Can you work these out from the model? Positions are in its coordinate system, mm. A direction names the side the tool comes from. Coordinates: 2 decimals unless noted, no trailing zeros. Write each loop counter-clockwise with the first axis right and the second up, starting at its lowest first coordinate (ties: lowest second). Pieces come first, ordered by that corner, then holes. Notation, with made-up numbers: (57, -9.75) -> (91, -9.75) arc R19 ccw to (91, 16.25) -> close; hole circle Ø6 at (42, -26.5). An arc over 180 degrees is marked (long way). Use one line per item in the form item = value.
```python
from build123d import *

# Parameters (mm, degrees)
EXTRUDE_1_DEPTH              = 4
HOLE_WIZARD_M5_1_D           = 8
HOLE_WIZARD_M5_1_DEPTH       = 12.4
HOLE_WIZARD_M5_1_CBORE_D     = 9.5
HOLE_WIZARD_M5_1_CBORE_DEPTH = 0.9
HOLE_WIZARD_M5_1_TIP         = 2.403442476
HOLE_WIZARD_M5_2_D           = 8
HOLE_WIZARD_M5_2_DEPTH       = 12.4
HOLE_WIZARD_M5_2_CBORE_D     = 9.5
HOLE_WIZARD_M5_2_CBORE_DEPTH = 0.9
HOLE_WIZARD_M5_2_TIP         = 2.403442476


with BuildPart() as part:
    # 草图2 → 凸台-拉伸1 (new body)
    with BuildSketch(Plane(origin=(0, 0, 0), x_dir=(1, 0, 0), z_dir=(0, 1, 0))):
        with BuildLine():
            Line((20, 21.641016151), (28.741669751, 6.5))
            Line((28.741669751, 6.5), (40, 6.5))
            ThreePointArc((40, 6.5), (43.25, 5.629165125), (45.629165125, 3.25))
            Line((45.629165125, 3.25), (25.629165125, 37.891016151))
            ThreePointArc((25.629165125, 37.891016151), (26.5, 34.641016151), (25.629165125, 31.391016151))
            Line((25.629165125, 31.391016151), (20, 21.641016151))
        make_face()
        with BuildLine():
            Line((28.741669751, 6.5), (11.258330249, 6.5))
            Line((11.258330249, 6.5), (5.629165125, -3.25))
            ThreePointArc((5.629165125, -3.25), (3.25, -5.629165125), (0, -6.5))
            Line((0, -6.5), (40, -6.5))
            ThreePointArc((40, -6.5), (36.75, -5.629165125), (34.370834875, -3.25))
            Line((34.370834875, -3.25), (28.741669751, 6.5))
        make_face()
        with BuildLine():
            Line((40, 6.5), (28.741669751, 6.5))
            Line((28.741669751, 6.5), (34.370834875, -3.25))
            ThreePointArc((34.370834875, -3.25), (36.75, -5.629165125), (40, -6.5))
            ThreePointArc((40, -6.5), (45.629165125, -3.25), (45.629165125, 3.25))
            ThreePointArc((45.629165125, 3.25), (43.25, 5.629165125), (40, 6.5))
        make_face()
        with BuildLine():
            ThreePointArc((-5.629165125, 3.25), (-3.25, 5.629165125), (0, 6.5))
            Line((0, 6.5), (11.258330249, 6.5))
            Line((11.258330249, 6.5), (20, 21.641016151))
            Line((20, 21.641016151), (14.370834875, 31.391016151))
            ThreePointArc((14.370834875, 31.391016151), (13.5, 34.641016151), (14.370834875, 37.891016151))
            Line((14.370834875, 37.891016151), (-5.629165125, 3.25))
        make_face()
        with BuildLine():
            Line((14.370834875, 31.391016151), (20, 21.641016151))
            Line((20, 21.641016151), (25.629165125, 31.391016151))
            ThreePointArc((25.629165125, 31.391016151), (26.5, 34.641016151), (25.629165125, 37.891016151))
            ThreePointArc((25.629165125, 37.891016151), (20, 41.141016151), (14.370834875, 37.891016151))
            ThreePointArc((14.370834875, 37.891016151), (13.5, 34.641016151), (14.370834875, 31.391016151))
        make_face()
        with BuildLine():
            Line((11.258330249, 6.5), (0, 6.5))
            ThreePointArc((0, 6.5), (-3.25, 5.629165125), (-5.629165125, 3.25))
            ThreePointArc((-5.629165125, 3.25), (-5.629165125, -3.25), (0, -6.5))
            ThreePointArc((0, -6.5), (3.25, -5.629165125), (5.629165125, -3.25))
            Line((5.629165125, -3.25), (11.258330249, 6.5))
        make_face()
        Polygon((20, 21.641016151), (11.258330249, 6.5), (28.741669751, 6.5), align=None)
    extrude(amount=EXTRUDE_1_DEPTH)

    # M5 六角头螺栓的柱形沉头孔1
    with Locations(Plane(origin=(0, 4, 0), x_dir=(1, 0, 0), z_dir=(0, 1, 0))):
        with Locations((0, 0)):
            CounterBoreHole(HOLE_WIZARD_M5_1_D / 2, HOLE_WIZARD_M5_1_CBORE_D / 2, HOLE_WIZARD_M5_1_CBORE_DEPTH, depth=HOLE_WIZARD_M5_1_DEPTH)
            with Locations((0, 0, -(HOLE_WIZARD_M5_1_DEPTH + HOLE_WIZARD_M5_1_TIP / 2))):  # 118° drill point
                Cone(0, HOLE_WIZARD_M5_1_D / 2, HOLE_WIZARD_M5_1_TIP, mode=Mode.SUBTRACT)

    # M5 六角头螺栓的柱形沉头孔2
    with Locations(Plane(origin=(0, 0, 0), x_dir=(-1, 0, 0), z_dir=(0, -1, 0))):
        with Locations((-40, 0), (-20, 34.641016151)):
            CounterBoreHole(HOLE_WIZARD_M5_2_D / 2, HOLE_WIZARD_M5_2_CBORE_D / 2, HOLE_WIZARD_M5_2_CBORE_DEPTH, depth=HOLE_WIZARD_M5_2_DEPTH)
            with Locations((0, 0, -(HOLE_WIZARD_M5_2_DEPTH + HOLE_WIZARD_M5_2_TIP / 2))):  # 118° drill point
                Cone(0, HOLE_WIZARD_M5_2_D / 2, HOLE_WIZARD_M5_2_TIP, mode=Mode.SUBTRACT)


solid = part.part
```
Q1. For faces 1 (the flat face through (20, 0, -12)), 2 (the cylindrical face through (2.192, 3.556, 4.214)), 3 (the flat face through (44, 0.9, 2)), which set-ups out of +Z, -Z, +X, -X, +Y, -Y let a thin tool reach every point of the face, with its end or its side?
Return value:
face_1 = +Z, -Z, +X, -X, -Y
face_2 = +Y
face_3 = -Y
Q2. Suppose I cut it at D-D (z = -36.5). Write out the boundary of the cut face in (x, y).
Return value:
outline = (13.57, 0) -> (15.63, 0) -> (15.63, 0.9) -> (16.46, 0.9) -> (16.46, 4) -> (13.57, 4) -> close; (23.54, 0.9) -> (24.37, 0.9) -> (24.37, 0) -> (26.43, 0) -> (26.43, 4) -> (23.54, 4) -> close
Q3. Thinking about a two-plate mould opening in Z: for faces 4 (the cylindrical face through (0.867, 1.528, 3.905)), 5 (the flat face through (20, 2, 6.5)), 6 (the cylindrical face through (45.6, 2, 3.3)), 7 (the flat face through (-4, 3.1, 2)), which applies, released by +Z, released by -Z, zero draft, split by the parting line, or undercut?
Return value:
face_4 = undercut
face_5 = released by +Z
face_6 = split by the parting line
face_7 = undercut
Q4. Will these pins go through, and if not, where does the flat tip stop? pin 1 (3 mm diameter, centred on x = 32.5, z = -12.5, fed in from -Y); pin 2 (1.5 mm diameter, centred on y = 1, z = -2, fed in from -X); pin 3 (9 mm diameter, centred on x = 0, z = 0, fed in from +Y); pin 4 (9 mm diameter, centred on x = 40, z = 0, fed in from -Y).
Return value:
pin_1 = 0
pin_2 = -6.38
pin_3 = 3.1
pin_4 = 0.9
Q5. Suppose I cut it at A-A (x = 20). Write out the boundary of the cut face in (y, z), then the cut area to 3 significant figures.
Return value:
outline = (0, -41.14) -> (4, -41.14) -> (4, -38.64) -> (0.9, -38.64) -> (0.9, -39.39) -> (0, -39.39) -> close; (0, -29.89) -> (0.9, -29.89) -> (0.9, -30.64) -> (4, -30.64) -> (4, 6.5) -> (0, 6.5) -> close
area = 157 mm2
Q6. Suppose I cut it at B-B (z = 0). Write out the boundary of the cut face in (x, y).
Return value:
outline = (-6.5, 0) -> (-4, 0) -> (-4, 3.1) -> (-4.75, 3.1) -> (-4.75, 4) -> (-6.5, 4) -> close; (4, 0) -> (35.25, 0) -> (35.25, 0.9) -> (36, 0.9) -> (36, 4) -> (4.75, 4) -> (4.75, 3.1) -> (4, 3.1) -> close; (44, 0.9) -> (44.75, 0.9) -> (44.75, 0) -> (46.5, 0) -> (46.5, 4) -> (44, 4) -> close
Q7. Suppose I cut it at C-C (y = 2.4). Write out the boundary of the cut face in (x, z), then the cut area to 3 significant figures.
Return value:
outline = (-5.63, -3.25) -> (14.37, -37.89) arc R6.5 ccw to (25.63, -37.89) -> (45.63, -3.25) arc R6.5 ccw to (40, 6.5) -> (0, 6.5) arc R6.5 ccw to start; hole circle Ø8 at (0, 0); hole circle Ø8 at (20, -34.64); hole circle Ø8 at (40, 0)
area = 1,450 mm2
Q8. If I drill on line 1 (X direction, y = 2.35, z = -2); line 2 (Z direction, x = 20, y = 0.55); line 3 (Z direction, x = 0, y = 2.2), over which ranges is the centre line in solid material (lowest first)? Write a range as from..to.
Return value:
line_1 = -6.18..-3.46, 3.46..36.54, 43.46..46.18
line_2 = -41.14..-39.39, -29.89..6.5
line_3 = -13..-4, 4..6.5
